```python
from build123d import *

# Parameters (mm, degrees)
SKETCH1_W            = 30
SKETCH1_H            = 10
BOSS_EXTRUDE1_DEPTH  = 3
M3_CLEARANCE_HOLE1_D = 3.2
FILLET1_R            = 0.5


with BuildPart() as part:
    # Sketch1 → Boss-Extrude1 (new body)
    with BuildSketch(Plane.XY):
        Rectangle(SKETCH1_W, SKETCH1_H)
    extrude(amount=BOSS_EXTRUDE1_DEPTH)

    # M3 Clearance Hole1 (through all)
    with Locations(Plane.XY.offset(3)):
        with Locations((-11.5, 0), (11.5, 0)):
            Hole(M3_CLEARANCE_HOLE1_D / 2)

    # Fillet1
    fillet1_edges = [part.edges().sort_by_distance(p)[0] for p in [
        (-15, 5, 1.5),
        (15, 5, 1.5),
        (15, -5, 1.5),
        (-15, -5, 1.5),
    ]]
    fillet(fillet1_edges, radius=FILLET1_R)


solid = part.part
```
Geometry: final body of the model. Coordinates: model frame, mm. Coordinates: 2 decimals unless noted, no trailing zeros. Order: outer loops, then holes, each group sorted by start corner. A loop starts at its lowest first (then second) coordinate and runs counter-clockwise, first axis right, second up. Notation, with made-up numbers: M 41.25,26.25 L 49.25,26.25 A37 ccw 49.25,62.25 Z; hole C 25,78 d3. An arc over 180 degrees is marked long. Answer in a Markdown table with one row per item. Add a question column.
Q1. Section query B-B on z = 1.8. Return the cut outline in (x, y).
Q2. Mould query, pull axis X, two halves, no side actions, for faces 1 (the cylindrical face through (13.1, 0.07, 1.48)), 2 (the flat face through (15, 0, 1)), 3 (the flat face through (0, 5, 1)), 4 (the cylindrical face through (-9.9, 0.07, 1.48)). Classes: released by +X, released by -X, zero draft, split by the parting line, or undercut.
Q3. Section query C-C on x = -11.75. Return the cut outline in (y, z), and give its area (3 significant figures).
Q4. Section query A-A on y = 0. Return the cut outline in (x, z).
Q5. Contact query for a flat-ended pin moving along its axis: P1, Ø1.9, axis at x = 11.5, y = 0, coming from the -Z side. Output: stop coordinate, or through.
Q6. Line query: L1, parallel to Y at x = 11.5, z = 0.65; L2, parallel to X at y = -0.75, z = 2.35; L3, parallel to X at y = -1, z = 0.6. Output: solid intervals per line, ascending.
Completed:
| question | item | result |
|---|---|---|
| 1 | outline | M -15,-4.5 A0.5 ccw -14.5,-5 L 14.5,-5 A0.5 ccw 15,-4.5 L 15,4.5 A0.5 ccw 14.5,5 L -14.5,5 A0.5 ccw -15,4.5 Z; hole C -11.5,0 d3.2; hole C 11.5,0 d3.2 |
| 2 | face 1 | undercut |
| 2 | face 2 | released by +X |
| 2 | face 3 | zero draft |
| 2 | face 4 | undercut |
| 3 | outline | M -5,0 L -1.58,0 L -1.58,3 L -5,3 Z; M 1.58,0 L 5,0 L 5,3 L 1.58,3 Z |
| 3 | area | 20.5 mm2 |
| 4 | outline | M -15,0 L -13.1,0 L -13.1,3 L -15,3 Z; M -9.9,0 L 9.9,0 L 9.9,3 L -9.9,3 Z; M 13.1,0 L 15,0 L 15,3 L 13.1,3 Z |
| 5 | P1 | passes through |
| 6 | L1 | y = -5 to -1.6, 1.6 to 5 |
| 6 | L2 | x = -15 to -12.91, -10.09 to 10.09, 12.91 to 15 |
| 6 | L3 | x = -15 to -12.75, -10.25 to 10.25, 12.75 to 15 |
